For this review, take the finished solid that the model builds, in its own axes (mm). Round coordinates to 2 decimals unless told otherwise and drop trailing zeros. Order: outer loops, then holes, each group sorted by start corner. A loop starts at its lowest first (then second) coordinate and runs counter-clockwise, first axis right, second up.
Autodesk Fusion 360 part; units mm, degrees
sketch "Skizze1" plane through (0, 0, 0) normal (0, 1, 0) x (1, 0, 0)
  circle A0 centre (0, 0) radius 45
  dimension "d1" = 90
extrude "Extrusion1" add sketch "Skizze1" along normal blind 7
cylinder "Grundkörper Zylinder1" cut diameter 5.5 height -10 placed x (1, 0, 0) y (0, 0, -1) z (0, 1, 0) at (0, 7, 0)
cylinder "Grundkörper Zylinder2" cut diameter 10 height -5 placed x (1, 0, 0) y (0, 0, -1) z (0, 1, 0) at (0, 7, 0)
fillet "Abrundung1" radius 1 2 edges at (-41.9547, 0, 16.2727) (-41.9547, 7, 16.2727)
fillet "Abrundung2" radius 0.3 2 edges at (0.9944, 0, 2.5639) (0.9944, 2, 2.5639)
fillet "Abrundung3" radius 0.7 1 edges at (-1.8081, 7, 4.6616)
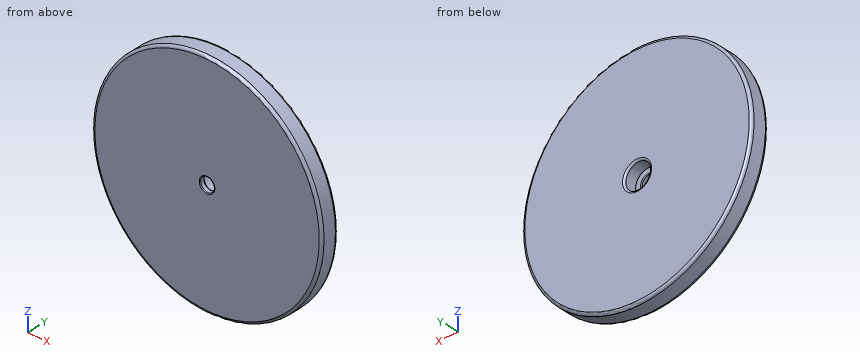
(1) Add section C-C on y = 3.5. Give the boundary of the cut face in (x, z), plus the area to 3 significant figures.
(2) Wall thickness on L1, parallel to Z at x = 0, y = 3.5; L2, parallel to X at y = 1.1, z = 0: over which ranges is each line inside the solid? List them lowest first.
(3) Add section A-A on x = 0. Give the boundary of the cut face in (y, z).
(4) Add section B-B on z = 0. Give the boundary of the cut face in (x, y).
(5) Clearance check with flat-ended pins moving along their axes: P1, Ø4, axis at y = 4, z = -22.5, coming from the -X side; P2, Ø5, axis at x = -0.5, z = 0.5, coming from the +Y side; P3, Ø2, axis at y = 2.5, z = 18, coming from the -X side; P4, Ø5, axis at x = 0, z = 0, coming from the -Y side. State where each tip first meets the part, or that it passes through.
Here are the results:
1. outline: circle Ø90 at (0, 0); hole circle Ø10 at (0, 0)
1. area: 6,280 mm2
2. L1: z = -45 to -5, 5 to 45
2. L2: x = -45 to -2.75, 2.75 to 45
3. outline: (0, -44) arc R1 ccw to (1, -45) - (6, -45) arc R1 ccw to (7, -44) - (7, -5.7) arc R0.7 ccw to (6.3, -5) - (2, -5) - (2, -3.05) arc R0.3 ccw to (1.7, -2.75) - (0.3, -2.75) arc R0.3 ccw to (0, -3.05) - close; (0, 3.05) arc R0.3 ccw to (0.3, 2.75) - (1.7, 2.75) arc R0.3 ccw to (2, 3.05) - (2, 5) - (6.3, 5) arc R0.7 ccw to (7, 5.7) - (7, 44) arc R1 ccw to (6, 45) - (1, 45) arc R1 ccw to (0, 44) - close
4. outline: (-45, 1) arc R1 ccw to (-44, 0) - (-3.05, 0) arc R0.3 ccw to (-2.75, 0.3) - (-2.75, 1.7) arc R0.3 ccw to (-3.05, 2) - (-5, 2) - (-5, 6.3) arc R0.7 ccw to (-5.7, 7) - (-44, 7) arc R1 ccw to (-45, 6) - close; (2.75, 0.3) arc R0.3 ccw to (3.05, 0) - (44, 0) arc R1 ccw to (45, 1) - (45, 6) arc R1 ccw to (44, 7) - (5.7, 7) arc R0.7 ccw to (5, 6.3) - (5, 2) - (3.05, 2) arc R0.3 ccw to (2.75, 1.7) - close
5. P1: stops at x = -40.06
5. P2: stops at y = 2
5. P3: stops at x = -41.67
5. P4: passes through
